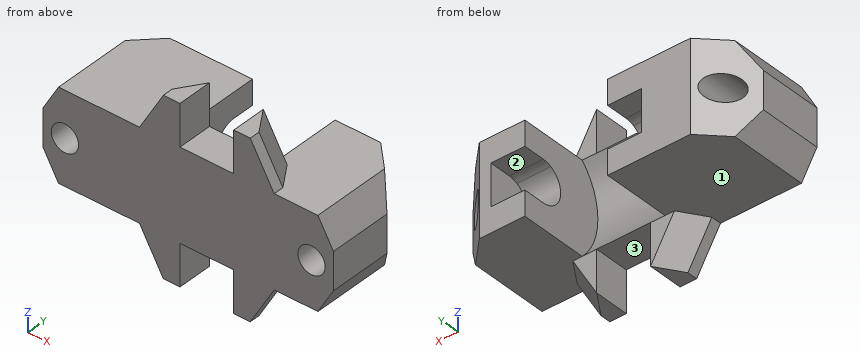
```python
from build123d import *
from OCP.BRepFilletAPI import BRepFilletAPI_MakeChamfer

# Parameters (mm, degrees)
SKIZZE1_R                       = 1.65
AUFSATZ_LINEAR_AUSTRAGEN1_DEPTH = 12.5
SCHNITT_LINEAR_START            = -10.3
SKIZZE2_R                       = 7.85
SKIZZE2_R_2                     = 2.5
SCHNITT_LINEAR_AUSTRAGEN1_DEPTH = 10
SCHNITT_LINEAR_START_2          = -5.3
SCHNITT_LINEAR_AUSTRAGEN2_DEPTH = 20
SCHNITT_LINEAR_AUSTRAGEN3_DEPTH = 4.5
SCHNITT_LINEAR_START_3          = -11
SCHNITT_LINEAR_AUSTRAGEN4_DEPTH = 11
AUFSATZ_LINEAR_START            = -4.248884
AUFSATZ_LINEAR_AUSTRAGEN2_DEPTH = 4.248884
FASE1_SIZE                      = 3
FASE1_SIZE2                     = 1.732050808
AUFSATZ_LINEAR_START_2          = 4.5
AUFSATZ_LINEAR_AUSTRAGEN3_DEPTH = 4.5
AUFSATZ_LINEAR_START_3          = 0.9
AUFSATZ_LINEAR_AUSTRAGEN4_DEPTH = 0.9
AUFSATZ_LINEAR_AUSTRAGEN5_DEPTH = 0.9


with BuildPart() as part:
    # Skizze1 → Aufsatz-Linear austragen1 (new body)
    with BuildSketch(Plane(origin=(0, 0, 0), x_dir=(1, 0, 0), z_dir=(0, 1, 0))):
        Polygon((0, 11), (-31.34722325, 11), (-33.223611625, 7.75), (-33.223611625, 3.25), (-31.34722325, 0), (0, 0), (1.876388375, 3.25), (1.876388375, 7.75), align=None)
        with Locations(Location((-0.773611625, 5.5, 0), (0, 0, 270))):
            Circle(SKIZZE1_R, mode=Mode.SUBTRACT)
        with Locations(Location((-30.573611625, 5.5, 0), (0, 0, 270))):
            Circle(SKIZZE1_R, mode=Mode.SUBTRACT)
    extrude(amount=AUFSATZ_LINEAR_AUSTRAGEN1_DEPTH)

    # Skizze2 → Schnitt-Linear austragen1 (cut)
    with BuildSketch(Plane(origin=(1.876388375, 0, 0), x_dir=(0, 0, -1), z_dir=(1, 0, 0)).offset(SCHNITT_LINEAR_START)):
        with Locations((5.5, 9.85)):
            Circle(SKIZZE2_R)
        with Locations((5.5, 9.85)):
            Circle(SKIZZE2_R_2, mode=Mode.SUBTRACT)
    extrude(amount=-SCHNITT_LINEAR_AUSTRAGEN1_DEPTH, mode=Mode.SUBTRACT)

    # Skizze3 → Schnitt-Linear austragen2 (cut)
    with BuildSketch(Plane(origin=(1.876388375, 0, 0), x_dir=(0, 0, -1), z_dir=(1, 0, 0)).offset(SCHNITT_LINEAR_START_2)):
        with BuildLine():
            Line((7.75, 12.5), (3.25, 12.5))
            Line((3.25, 12.5), (3.25, 10.939724736))
            ThreePointArc((3.25, 10.939724736), (5.5, 12.35), (7.75, 10.939724736))
            Line((7.75, 10.939724736), (7.75, 12.5))
        make_face()
        with BuildLine():
            Line((8, 12.5), (7.75, 12.5))
            Line((7.75, 12.5), (7.75, 10.939724736))
            ThreePointArc((7.75, 10.939724736), (7.936698586, 10.409016994), (8, 9.85))
            Line((8, 9.85), (8, 12.5))
        make_face()
        with BuildLine():
            Line((3.25, 12.5), (3, 12.5))
            Line((3, 12.5), (3, 9.85))
            ThreePointArc((3, 9.85), (3.063301414, 10.409016994), (3.25, 10.939724736))
            Line((3.25, 10.939724736), (3.25, 12.5))
        make_face()
        with BuildLine():
            ThreePointArc((7.75, 10.939724736), (5.5, 12.35), (3.25, 10.939724736))
            Line((3.25, 10.939724736), (3.25, 8.760275264))
            ThreePointArc((3.25, 8.760275264), (5.5, 7.35), (7.75, 8.760275264))
            Line((7.75, 8.760275264), (7.75, 10.939724736))
        make_face()
        with BuildLine():
            ThreePointArc((3.25, 10.939724736), (3.063301414, 10.409016994), (3, 9.85))
            ThreePointArc((3, 9.85), (3.063301414, 9.290983006), (3.25, 8.760275264))
            Line((3.25, 8.760275264), (3.25, 10.939724736))
        make_face()
        with BuildLine():
            ThreePointArc((8, 9.85), (7.936698586, 10.409016994), (7.75, 10.939724736))
            Line((7.75, 10.939724736), (7.75, 8.760275264))
            ThreePointArc((7.75, 8.760275264), (7.936698586, 9.290983006), (8, 9.85))
        make_face()
    extrude(amount=-SCHNITT_LINEAR_AUSTRAGEN2_DEPTH, mode=Mode.SUBTRACT)

    # Skizze4 → Schnitt-Linear austragen3 (cut)
    with BuildSketch(Plane(origin=(-23.423611625, 0, 0), x_dir=(0, 0, -1), z_dir=(1, 0, 0))):
        with BuildLine():
            Line((10.25, 12.5), (0.75, 12.5))
            Line((0.75, 12.5), (0.75, 9.85))
            ThreePointArc((0.75, 9.85), (5.5, 5.1), (10.25, 9.85))
            Line((10.25, 9.85), (10.25, 12.5))
        make_face()
    extrude(amount=-SCHNITT_LINEAR_AUSTRAGEN3_DEPTH, mode=Mode.SUBTRACT)

    # Skizze5 → Schnitt-Linear austragen4 (cut)
    with BuildSketch(Plane.XY.offset(SCHNITT_LINEAR_START_3)):
        Polygon((1.876388375, 12.5), (-2.923611625, 12.5), (1.876388375, 7.7), align=None)
        Polygon((-33.223611625, 12.5), (-28.423611625, 12.5), (-33.223611625, 7.7), align=None)
    extrude(amount=SCHNITT_LINEAR_AUSTRAGEN4_DEPTH, mode=Mode.SUBTRACT)

    # Skizze6 → Aufsatz-Linear austragen2 (add)
    with BuildSketch(Plane.XZ.offset(AUFSATZ_LINEAR_START)):
        Polygon((-16.673611625, 0), (-16.673611625, 5), (-18.673611625, 5), (-21.560362971, 0), align=None)
        Polygon((-10.173611625, 0), (-10.173611625, 5), (-8.173611625, 5), (-5.286860279, 0), align=None)
        Polygon((-18.673611625, -16), (-21.560362971, -11), (-16.673611625, -11), (-16.673611625, -16), align=None)
        Polygon((-10.173611625, -11), (-5.286860279, -11), (-8.173611625, -16), (-10.173611625, -16), align=None)
    extrude(amount=AUFSATZ_LINEAR_AUSTRAGEN2_DEPTH)

    # Fase1: one chamfer whose edges measure the first distance from different faces: ONE call of the kernel's chamfer builder (chamfer() names one face for all edges)
    fase1_edges_1 = [part.edges().sort_by_distance(p)[0] for p in [
        (-6.730235952, 4.248884, -13.5),
    ]]
    fase1_side_1 = [part.faces().sort_by_distance(p)[0] for p in [
        (-6.730235952, 2.124442, -13.5),
    ]]
    fase1_edges_2 = [part.edges().sort_by_distance(p)[0] for p in [
        (-20.116987298, 4.248884, -13.5),
    ]]
    fase1_side_2 = [part.faces().sort_by_distance(p)[0] for p in [
        (-20.116987298, 2.124442, -13.5),
    ]]
    fase1_edges_3 = [part.edges().sort_by_distance(p)[0] for p in [
        (-6.730235952, 4.248884, 2.5),
    ]]
    fase1_side_3 = [part.faces().sort_by_distance(p)[0] for p in [
        (-6.730235952, 2.124442, 2.5),
    ]]
    fase1_edges_4 = [part.edges().sort_by_distance(p)[0] for p in [
        (-20.116987298, 4.248884, 2.5),
    ]]
    fase1_side_4 = [part.faces().sort_by_distance(p)[0] for p in [
        (-20.116987298, 2.124442, 2.5),
    ]]
    fase1 = BRepFilletAPI_MakeChamfer(part.part.solid().wrapped)
    for e in fase1_edges_1:
        fase1.Add(FASE1_SIZE, FASE1_SIZE2, e.wrapped, fase1_side_1[0].wrapped)  # the first distance lies on this face
    for e in fase1_edges_2:
        fase1.Add(FASE1_SIZE, FASE1_SIZE2, e.wrapped, fase1_side_2[0].wrapped)  # the first distance lies on this face
    for e in fase1_edges_3:
        fase1.Add(FASE1_SIZE, FASE1_SIZE2, e.wrapped, fase1_side_3[0].wrapped)  # the first distance lies on this face
    for e in fase1_edges_4:
        fase1.Add(FASE1_SIZE, FASE1_SIZE2, e.wrapped, fase1_side_4[0].wrapped)  # the first distance lies on this face
    add(Compound.cast(fase1.Shape()), mode=Mode.REPLACE)

    # Skizze7 → Aufsatz-Linear austragen3 (add)
    with BuildSketch(Plane(origin=(-27.923611625, 0, 0), x_dir=(0, 0, -1), z_dir=(1, 0, 0)).offset(AUFSATZ_LINEAR_START_2)):
        with BuildLine():
            Line((10.25, 12.5), (0.75, 12.5))
            Line((0.75, 12.5), (0.75, 9.85))
            ThreePointArc((0.75, 9.85), (5.5, 5.1), (10.25, 9.85))
            Line((10.25, 9.85), (10.25, 12.5))
        make_face()
    extrude(amount=-AUFSATZ_LINEAR_AUSTRAGEN3_DEPTH)

    # Skizze8 → Aufsatz-Linear austragen4 (add)
    with BuildSketch(Plane(origin=(-23.423611625, 0, 0), x_dir=(0, 0, -1), z_dir=(1, 0, 0)).offset(AUFSATZ_LINEAR_START_3)):
        with BuildLine():
            Line((8, 12.5), (3, 12.5))
            Line((3, 12.5), (3, 9.85))
            ThreePointArc((3, 9.85), (5.5, 7.35), (8, 9.85))
            Line((8, 9.85), (8, 12.5))
        make_face()
    extrude(amount=-AUFSATZ_LINEAR_AUSTRAGEN4_DEPTH)

    # Skizze9 → Aufsatz-Linear austragen5 (add)
    with BuildSketch(Plane.ZY.offset(3.423611625)):
        with BuildLine():
            Line((-3, 9.85), (-3, 12.5))
            Line((-3, 12.5), (-8, 12.5))
            Line((-8, 12.5), (-8, 9.85))
            ThreePointArc((-8, 9.85), (-5.5, 7.35), (-3, 9.85))
        make_face()
    extrude(amount=AUFSATZ_LINEAR_AUSTRAGEN5_DEPTH)


solid = part.part
```
The listing builds one solid part. Answer for the finished solid, in the listing's coordinates (mm). Face numbers are marked on the shaded views. A direction names the side the tool comes from. Give positions to 0.01 mm unless a question says otherwise; leave off trailing zeros. Loops run counter-clockwise (first coordinate to the right, second up) from the corner with the lowest first, then second, coordinate; pieces in that order, holes last. Notation, with made-up numbers: (48, -19) - (84, -19) arc R24 ccw to (84, 4) - close; hole circle Ø8 at (42.5, 46). An arc over 180 degrees is marked (long way). Answer as CSV lines item,"result". Start each with the question number.
Item 1: A cutting plane is placed at C-C on y = 3.25. Count the separate pieces of the cut face and the enclosed holes in it, then the cut area to 3 significant figures.
Item 2: For the marked faces 1, 2 and 3, determine the directions among +Z, -Z, +X, -X, +Y, -Y from which every point of the face is accessible in a straight line to the end or side of a thin tool.
Item 3: A cutting plane is placed at D-D on x = -1.5. Determine the outline of the cut face in (y, z).
Item 4: A cutting plane is placed at A-A on z = -5.5. Determine the outline of the cut face in (x, y), then the cut area to 3 significant figures.
Item 5: A cutting plane is placed at B-B on z = -13.75. Determine the outline of the cut face in (x, y).
Item 6: Find the intervals of material crossed by line 1 (X direction, y = 3.25, z = -5.5); line 2 (X direction, y = 12, z = -2); line 3 (Z direction, x = -4, y = 3.5), in increasing order. Write a range as from..to.
Item 7: Each of these flat-tipped pins is pushed along its axis until it touches: pin 1 (6 mm diameter, centred on x = -28, y = 3.5, fed in from +Z); pin 2 (3.5 mm diameter, centred on y = 2, z = -14, fed in from -X); pin 3 (2 mm diameter, centred on x = -4, z = 1.5, fed in from +Y); pin 4 (2.5 mm diameter, centred on x = -9.5, z = 3, fed in from +Y). Where does it stop, or does it pass through?
Found:
1,separate pieces,"1"
1,enclosed holes,"3"
1,area,"314 mm^2"
2,face 1,"-Z, -X, +Y"
2,face 2,"+Y"
2,face 3,"-Z, +Y, -Y"
3,outline,"(0, -11) - (11.08, -11) - (11.08, -6.98) - (0, -6.98) - close; (0, -4.02) - (11.08, -4.02) - (11.08, 0) - (0, 0) - close"
4,outline,"(-33.22, 0) - (-32.22, 0) - (-32.22, 8.7) - (-33.22, 7.7) - close; (-28.92, 0) - (-2.42, 0) - (-2.42, 12) - (-2.92, 12.5) - (-4.32, 12.5) - (-4.32, 7.35) - (-8.42, 7.35) - (-8.42, 2) - (-18.42, 2) - (-18.42, 7.35) - (-22.52, 7.35) - (-22.52, 12.5) - (-28.42, 12.5) - (-28.92, 12) - close; (0.88, 0) - (1.88, 0) - (1.88, 7.7) - (0.88, 8.7) - close"
4,area,"200 mm^2"
5,outline,"(-19.97, 0) - (-16.67, 0) - (-16.67, 4.25) - (-17.97, 4.25) - (-19.97, 1.25) - close; (-10.17, 0) - (-6.87, 0) - (-6.87, 1.25) - (-8.87, 4.25) - (-10.17, 4.25) - close"
6,line 1,"x = -33.22..-32.22, -28.92..-18.42, -8.42..-2.42, 0.88..1.88"
6,line 2,"x = -28.92..-18.42, -8.42..-2.42"
6,line 3,"z = -11..0"
7,pin 1,"stops at z = 0"
7,pin 2,"stops at x = -20.74"
7,pin 3,"passes through"
7,pin 4,"stops at y = 4.25"
